from build123d import *

# Parameters (mm, degrees)
SKETCH_1_W          = 60
SKETCH_1_H          = 60
EXTRUDE_1_DEPTH     = 10
SKETCH_3_R          = 30
EXTRUDE_2_DEPTH     = 37
SKETCH_4_W          = 60
SKETCH_4_H          = 60
EXTRUDE_3_DEPTH     = 32
SKETCH_5_R          = 25
EXTRUDE_4_DEPTH     = 3
SKETCH_6_R          = 8.5
EXTRUDE_5_DEPTH     = 2
SKETCH_7_R          = 7
EXTRUDE_6_DEPTH     = 30
SKETCH_8_R          = 7
CUT_EXTRUDE_1_DEPTH = 30
SKETCH_9_R          = 2.75
CUT_EXTRUDE_2_DEPTH = 30
CUT_EXTRUDE_3_DEPTH = 3


with BuildPart() as part:
    # 草图1 → 拉伸1 (new body)
    with BuildSketch(Plane.XY):
        with Locations((30, -30)):
            Rectangle(SKETCH_1_W, SKETCH_1_H)
    extrude(amount=EXTRUDE_1_DEPTH)

    # 草图3 → 拉伸2 (add)
    with BuildSketch(Plane.XY.offset(10)):
        with Locations((30, -30)):
            Circle(SKETCH_3_R)
    extrude(amount=EXTRUDE_2_DEPTH)

    # 草图4 → 拉伸3 (add)
    with BuildSketch(Plane.XY.offset(47)):
        with Locations((30, -30)):
            Rectangle(SKETCH_4_W, SKETCH_4_H)
    extrude(amount=EXTRUDE_3_DEPTH)

    # 草图5 → 拉伸4 (add)
    with BuildSketch(Plane(origin=(0, 0, 0), x_dir=(-1, 0, 0), z_dir=(0, 0, -1))):
        with Locations(Location((-30, -30, 0), (0, 0, 180))):
            Circle(SKETCH_5_R)
    extrude(amount=EXTRUDE_4_DEPTH)

    # 草图6 → 拉伸5 (add)
    with BuildSketch(Plane(origin=(0, 0, -3), x_dir=(-1, 0, 0), z_dir=(0, 0, -1))):
        with Locations((-30, -30)):
            Circle(SKETCH_6_R)
    extrude(amount=EXTRUDE_5_DEPTH)

    # 草图7 → 拉伸6 (add)
    with BuildSketch(Plane(origin=(0, 0, -5), x_dir=(-1, 0, 0), z_dir=(0, 0, -1))):
        with Locations((-30, -30)):
            Circle(SKETCH_7_R)
    extrude(amount=EXTRUDE_6_DEPTH)

    # 草图8 → 切除-拉伸1 (cut)
    with BuildSketch(Plane.XY.offset(79)):
        with Locations(Location((30, -30, 0), (0, 0, 180))):
            Circle(SKETCH_8_R)
    extrude(amount=-CUT_EXTRUDE_1_DEPTH, mode=Mode.SUBTRACT)

    # 草图9 → 切除-拉伸2 (cut)
    with BuildSketch(Plane(origin=(0, 0, 0), x_dir=(-1, 0, 0), z_dir=(0, 0, -1))):
        with Locations((-5.251262658, -5.251262658)):
            Circle(SKETCH_9_R)
        with Locations((-5.251262658, -54.748737342)):
            Circle(SKETCH_9_R)
        with Locations((-54.748737342, -54.748737342)):
            Circle(SKETCH_9_R)
        with Locations((-54.748737342, -5.251262658)):
            Circle(SKETCH_9_R)
    extrude(amount=-CUT_EXTRUDE_2_DEPTH, mode=Mode.SUBTRACT)

    # 草图10 → 切除-拉伸3 (cut)
    with BuildSketch(Plane(origin=(0, -23, 0), x_dir=(-1, 0, 0), z_dir=(0, 1, 0))):
        with BuildLine():
            Line((-32.5, -10), (-32.5, -30))
            ThreePointArc((-32.5, -30), (-30, -32.5), (-27.5, -30))
            Line((-27.5, -30), (-27.5, -10))
            ThreePointArc((-27.5, -10), (-30, -7.5), (-32.5, -10))
        make_face()
    extrude(amount=-CUT_EXTRUDE_3_DEPTH, mode=Mode.SUBTRACT)


solid = part.part
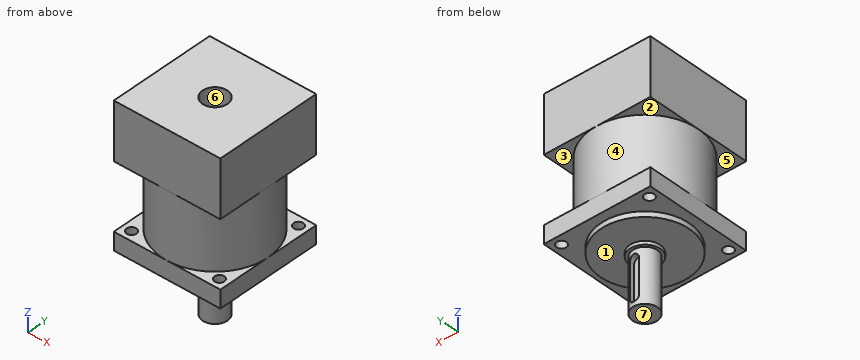
Read the model definition and answer for the solid it produces. Units are mm, in the model's axes. Face numbers are marked on the shaded views. A direction names the side the tool comes from. Round coordinates to 2 decimals unless told otherwise and drop trailing zeros. Write each loop counter-clockwise with the first axis right and the second up, starting at its lowest first coordinate (ties: lowest second). Pieces come first, ordered by that corner, then holes.
1. Given pin 1 Ø1.3 at (y, z) = (-25, -19.5) entering from +X; pin 2 Ø15 at (x, y) = (11.5, -50) entering from -Z; pin 3 Ø3 at (y, z) = (-24, -21.5) entering from -X, each flat-ended and moving along its own axis, determine where each tip first touches the part or whether it passes through.
2. Which of the six approach directions +Z, -Z, +X, -X, +Y, -Y give full straight-line access (tool end or side, diameter ignored) to the marked faces 1, 2, 3 and 4?
3. The part is cut by section B-B, the plane y = -53.5. Determine the outline of the cut face in (x, z).
4. The part is cut by section D-D, the plane y = -32. Determine the outline of the cut face in (x, z), then the cut area to 3 significant figures.
5. Straight lines are drawn through the part: L1, parallel to X at y = -30, z = 57.75; L2, parallel to X at y = -4.5, z = 1.5; L3, parallel to Z at x = 12.5, y = -4.5. For each, find the intervals that lie inside material, in ascending order.
6. The part is cut by section A-A, the plane z = 51. Determine the outline of the cut face in (x, y), then the cut area to 3 significant figures.
7. The part is cut by section C-C, the plane x = 24.5. Determine the outline of the cut face in (y, z), then the cut area to 3 significant figures.
8. Determine the mould class of the marked faces 5, 6 and 7 for opening direction Z: pulls with the +Z half, pulls with the -Z half, needs draft (parallel to the pull), parting line crosses it, or undercut.
Values:
1. pin 1: stops at x = 35.48
1. pin 2: stops at z = -3
1. pin 3: stops at x = 24.64
2. face 1: -Z
2. face 2: -X, +Y
2. face 3: +X, +Y
2. face 4: none
3. outline: (0, 0) - (2.8, 0) - (2.8, 10) - (0, 10) - close; (0, 47) - (11.35, 47) - (11.35, 10) - (7.7, 10) - (7.7, 0) - (21.47, 0) - (21.47, -3) - (38.53, -3) - (38.53, 0) - (52.3, 0) - (52.3, 10) - (48.65, 10) - (48.65, 47) - (60, 47) - (60, 79) - (0, 79) - close; (57.2, 0) - (60, 0) - (60, 10) - (57.2, 10) - close
4. outline: (0, 0) - (5.08, 0) - (5.08, -3) - (21.74, -3) - (21.74, -5) - (23.29, -5) - (23.29, -35) - (36.71, -35) - (36.71, -5) - (38.26, -5) - (38.26, -3) - (54.92, -3) - (54.92, 0) - (60, 0) - (60, 10) - (59.93, 10) - (59.93, 47) - (60, 47) - (60, 79) - (36.71, 79) - (36.71, 49) - (23.29, 49) - (23.29, 79) - (0, 79) - (0, 47) - (0.07, 47) - (0.07, 10) - (0, 10) - close
4. area: 4,920 mm2
5. L1: x = 0 to 23, 37 to 60
5. L2: x = 0 to 2.61, 7.9 to 52.1, 57.39 to 60
5. L3: z = 0 to 10, 47 to 79
6. outline: (0, -60) - (60, -60) - (60, 0) - (0, 0) - close; hole circle Ø14 at (30, -30)
6. area: 3,450 mm2
7. outline: (-60, 0) - (-54.39, 0) - (-54.39, -3) - (-36.48, -3) - (-36.48, -5) - (-34.33, -5) - (-34.33, -35) - (-25.67, -35) - (-25.67, -5) - (-23.52, -5) - (-23.52, -3) - (-5.61, -3) - (-5.61, 0) - (0, 0) - (0, 10) - (-0.51, 10) - (-0.51, 47) - (0, 47) - (0, 79) - (-25.67, 79) - (-25.67, 49) - (-34.33, 49) - (-34.33, 79) - (-60, 79) - (-60, 47) - (-59.49, 47) - (-59.49, 10) - (-60, 10) - close
7. area: 4,870 mm2
8. face 5: undercut
8. face 6: needs draft
8. face 7: pulls with the -Z half
